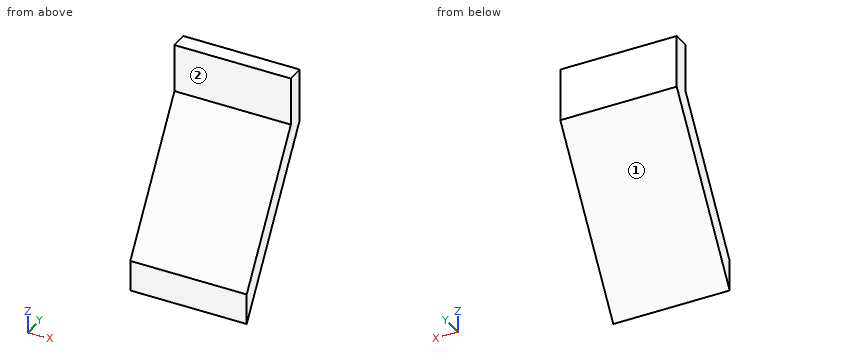
from build123d import *

# Parameters (mm, degrees)
CROQUIS2_W                 = 43
CROQUIS2_H                 = 30
SALIENTE_EXTRUIR1_DEPTH    = 30
CROQUIS3_W                 = 42.529407755
CROQUIS3_H                 = 25.558495791
CORTAR_EXTRUIR1_DEPTH      = 30
CORTAR_EXTRUIR2_START      = -7.5
CORTAR_EXTRUIR2_DEPTH      = 15
CORTAR_EXTRUIR4_DEPTH      = 4.5
CORTAR_EXTRUIR5_DEPTH      = 4.5
REDONDEO1_R                = 3
CROQUIS8_W                 = 15
CROQUIS8_H                 = 32.397186909
CORTAR_EXTRUIR6_DEPTH      = 4.5
CROQUIS9_W                 = 120.283196461
CROQUIS9_H                 = 78.810135234
CORTAR_EXTRUIR7_DEPTH      = 22.5
CORTAR_EXTRUIR9_DEPTH      = 22.5
CORTAR_EXTRUIR9_DEPTH_BACK = 29.5


with BuildPart() as part:
    # Croquis2 → Saliente-Extruir1 (new body)
    with BuildSketch(Plane(origin=(0, 0, 0), x_dir=(0, 0, -1), z_dir=(1, 0, 0))):
        with Locations((-19.783269962, -13.522813688)):
            Rectangle(CROQUIS2_W, CROQUIS2_H)
    extrude(amount=SALIENTE_EXTRUIR1_DEPTH)

    # Croquis3 → Cortar-Extruir1 (cut)
    with BuildSketch(Plane(origin=(30, 0, 0), x_dir=(0, 0, -1), z_dir=(1, 0, 0))):
        with Locations((-17.018566085, -31.302061584)):
            Rectangle(CROQUIS3_W, CROQUIS3_H)
        Polygon((-31.675073764, 1.477186312), (-3.283269962, -16.522813688), (1.716730038, -16.522813688), (1.716730038, 1.477186312), align=None)
    extrude(amount=-CORTAR_EXTRUIR1_DEPTH, mode=Mode.SUBTRACT)

    # Croquis4 → Cortar-Extruir2 (cut)
    with BuildSketch(Plane(origin=(30, 0, 0), x_dir=(0, 0, -1), z_dir=(1, 0, 0)).offset(CORTAR_EXTRUIR2_START)):
        Polygon((-41.283269962, -1.522813688), (-32.545919554, -1.522813688), (-8.886083053, -16.522813688), (-41.283269962, -16.522813688), align=None)
    extrude(amount=-CORTAR_EXTRUIR2_DEPTH, mode=Mode.SUBTRACT)

    # Croquis5 → Cortar-Extruir4 (cut)
    with BuildSketch(Plane(origin=(30, 0, 0), x_dir=(0, 0, -1), z_dir=(1, 0, 0))):
        Polygon((-3.283269962, -16.522813688), (-41.283269962, -16.522813688), (-41.283269962, 1.477186312), (-31.675073764, 1.477186312), align=None)
    extrude(amount=-CORTAR_EXTRUIR4_DEPTH, mode=Mode.SUBTRACT)

    # Croquis6 → Cortar-Extruir5 (cut)
    with BuildSketch(Plane.ZY):
        Polygon((3.283269962, -16.522813688), (41.283269962, -16.522813688), (41.283269962, 1.477186312), (31.675073764, 1.477186312), align=None)
    extrude(amount=-CORTAR_EXTRUIR5_DEPTH, mode=Mode.SUBTRACT)

    # Redondeo1
    redondeo1_edges = [part.edges().sort_by_distance(p)[0] for p in [
        (0, -17.522813688, -1.716730038),
        (30, -17.522813688, -1.716730038),
    ]]
    fillet(redondeo1_edges, radius=REDONDEO1_R)

    # Croquis8 → Cortar-Extruir6 (cut)
    with BuildSketch(Plane(origin=(0, -16.522813688, 0), x_dir=(1, 0, 0), z_dir=(0, 1, 0))):
        with Locations((15, -25.084676508)):
            Rectangle(CROQUIS8_W, CROQUIS8_H)
    extrude(amount=-CORTAR_EXTRUIR6_DEPTH, mode=Mode.SUBTRACT)

    # Croquis9 → Cortar-Extruir7 (cut)
    with BuildSketch(Plane.XZ.offset(18.522813688)):
        with Locations((17.6156444, 62.089659259)):
            Rectangle(CROQUIS9_W, CROQUIS9_H)
    extrude(amount=CORTAR_EXTRUIR7_DEPTH, mode=Mode.SUBTRACT)

    # Croquis10 → Cortar-Extruir9 (cut, two sides)
    with BuildSketch(Plane(origin=(25.5, 0, 0), x_dir=(0, 0, -1), z_dir=(1, 0, 0))) as cortar_extruir9_sk:
        Polygon((-41.283269962, -1.522813688), (-32.545919554, -1.522813688), (-8.886083053, -16.522813688), (1.716730038, -16.522813688), (18.108947867, -28.45757264), (-61.799912443, -25.241788427), align=None)
    extrude(amount=CORTAR_EXTRUIR9_DEPTH, mode=Mode.SUBTRACT)
    extrude(cortar_extruir9_sk.sketch, amount=-CORTAR_EXTRUIR9_DEPTH_BACK, mode=Mode.SUBTRACT)


solid = part.part
Can you work these out from the model? Positions are in its coordinate system, mm. Face numbers are marked on the shaded views. A direction names the side the tool comes from. Give positions to 0.01 mm unless a question says otherwise; leave off trailing zeros. Write each loop counter-clockwise with the first axis right and the second up, starting at its lowest first coordinate (ties: lowest second). Pieces come first, ordered by that corner, then holes. Notation, with made-up numbers: M -30.5,-35 L -5.5,-35 A9 ccw -5.5,-30 Z; hole C -11,-5 d4. An arc over 180 degrees is marked long. Answer in a Markdown table with one row per item. Add a question column.
Item 1: Imagine slicing it at B-B, the plane y = -0.25. Write out the boundary of the cut face in (x, z), plus the area to 3 significant figures.
Item 2: On a 3-axis mill with a long thin cutter (end or side, diameter ignored), from which of +Z, -Z, +X, -X, +Y, -Y can I reach the whole of each face in a straight line? I mean the marked faces 1 and 2. Say none if no direction works.
Item 3: For pin 1 Ø1.5 at (x, z) = (12.5, 10.5) entering from +Y; pin 2 Ø4 at (x, y) = (7, -11.5) entering from +Z; pin 3 Ø4.5 at (x, z) = (11, 36.5) entering from -Y; pin 4 Ø1.5 at (y, z) = (-7, 28.5) entering from +X, each with a flat end and sliding along its axis, tell me the tip position at first contact or that it passes through.
Item 4: Imagine slicing it at C-C, the plane z = 8.5. Write out the boundary of the cut face in (x, y).
Item 5: Imagine slicing it at A-A, the plane x = 19.25. Write out the boundary of the cut face in (y, z), plus the area to 3 significant figures.
Item 6: Please list where these lines run through material, in increasing order: L1, parallel to Y at x = 6.25, z = 39; L2, parallel to Z at x = 6.5, y = -0.25; L3, parallel to Y at x = 19.75, z = 20.5.
Evaluation:
| question | item | result |
|---|---|---|
| 1 | outline | M 4.5,28.95 L 25.5,28.95 L 25.5,41.28 L 4.5,41.28 Z |
| 1 | area | 259 mm² |
| 2 | face 1 | -Z, +X, -X, +Y |
| 2 | face 2 | +Z, +X, -X, -Y |
| 3 | pin 1 | stops at y = -11.47 |
| 3 | pin 2 | stops at z = 19.96 |
| 3 | pin 3 | stops at y = -1.52 |
| 3 | pin 4 | passes through |
| 4 | outline | M 4.5,-16.52 L 25.5,-16.52 L 25.5,-13.22 L 4.5,-13.22 Z |
| 5 | outline | M -16.52,3.28 L 1.48,31.68 L 1.48,41.28 L -1.52,41.28 L -1.52,32.55 L -16.52,8.89 Z |
| 5 | area | 120 mm² |
| 6 | L1 | y = -1.52 to 1.48 |
| 6 | L2 | z = 28.95 to 41.28 |
| 6 | L3 | y = -9.16 to -5.61 |
